```python
from build123d import *

# Parameters (mm, degrees)
F0_R      = 75.025987
F1_DEPTH  = 2148.84
F2_R      = 64.485043
F3_DEPTH  = 203.2
F3_FACE_R = 64.485043
F4_DEPTH  = 1513.84


with BuildPart() as f1:
    # F0 (on Right) → F1 (new body)
    with BuildSketch(Plane.YZ):
        Circle(F0_R)
    extrude(amount=F1_DEPTH)

    # F2 (on face) → F3 (cut)
    with BuildSketch(Plane.YZ.offset(2148.84)):
        Circle(F2_R)
    extrude(amount=-F3_DEPTH, mode=Mode.SUBTRACT)

    # F3_face (on face) → F4 (cut)
    with BuildSketch(Plane.YZ.offset(1945.64)):
        Circle(F3_FACE_R)
    extrude(amount=-F4_DEPTH, mode=Mode.SUBTRACT)


solid = f1.part
```
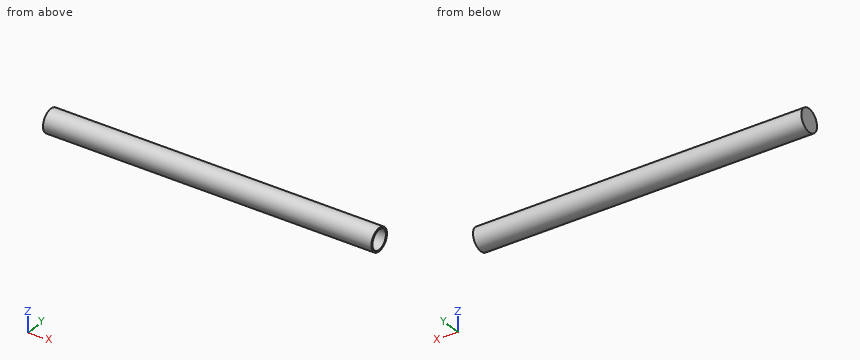
The model under review builds one solid part; all positions refer to its coordinate system, in mm. Give positions to 0.01 mm unless a question says otherwise; leave off trailing zeros. Write each loop counter-clockwise with the first axis right and the second up, starting at its lowest first coordinate (ties: lowest second). Pieces come first, ordered by that corner, then holes. Notation, with made-up numbers: (67.25, 38) - (120.25, 38) arc R37 ccw to (120.25, 77) - close; hole circle Ø8 at (62, -14.5). An arc over 180 degrees is marked (long way). Answer in a Markdown table with one row per item. Add a question column.
1. We need section C-C on x = 453. Write out the cut boundary in (y, z), then the cut area to 3 significant figures.
2. We need section A-A on y = 0. Write out the cut boundary in (x, z), then the cut area to 3 significant figures.
3. Insertion check: P1, Ø1.5, axis at x = 649, y = -58, coming from the +Z side; P2, Ø1.5, axis at x = 280, y = -15, coming from the +Z side; P3, Ø1.5, axis at x = 706, y = 25.5, coming from the +Z side; P4, Ø1, axis at y = -6.5, z = -8, coming from the -X side. Each pin has a flat end and moves straight along its axis. Give the tip position at first contact, or say it passes through.
4. Wall thickness on line 1 along Z through (x, y) = (1162.5, 0); line 2 along Y through (x, z) = (730.5, -5.5); line 3 along X through (y, z) = (-27, 48): over which ranges is each line inside the solid? List them lowest first. Write a range as [from, to].
Ans:
| question | item | result |
|---|---|---|
| 1 | outline | circle Ø150.05 at (0, 0); hole circle Ø128.97 at (0, 0) |
| 1 | area | 4,620 mm^2 |
| 2 | outline | (0, -75.03) - (2148.84, -75.03) - (2148.84, -64.49) - (431.8, -64.49) - (431.8, 64.49) - (2148.84, 64.49) - (2148.84, 75.03) - (0, 75.03) - close |
| 2 | area | 101,000 mm^2 |
| 3 | P1 | stops at z = 48.49 |
| 3 | P2 | stops at z = 73.66 |
| 3 | P3 | stops at z = 70.83 |
| 3 | P4 | stops at x = 0 |
| 4 | line 1 | z = [-75.03, -64.49], [64.49, 75.03] |
| 4 | line 2 | y = [-74.82, -64.25], [64.25, 74.82] |
| 4 | line 3 | x = [0, 431.8] |
